Input: dimensioned drawing with shaded views. Units: mm. Origin: part minimum x, y, z. Coordinates: 2 decimals unless noted, no trailing zeros. Order: outer loops, then holes, each group sorted by start corner. A loop starts at its lowest first (then second) coordinate and runs counter-clockwise, first axis right, second up.
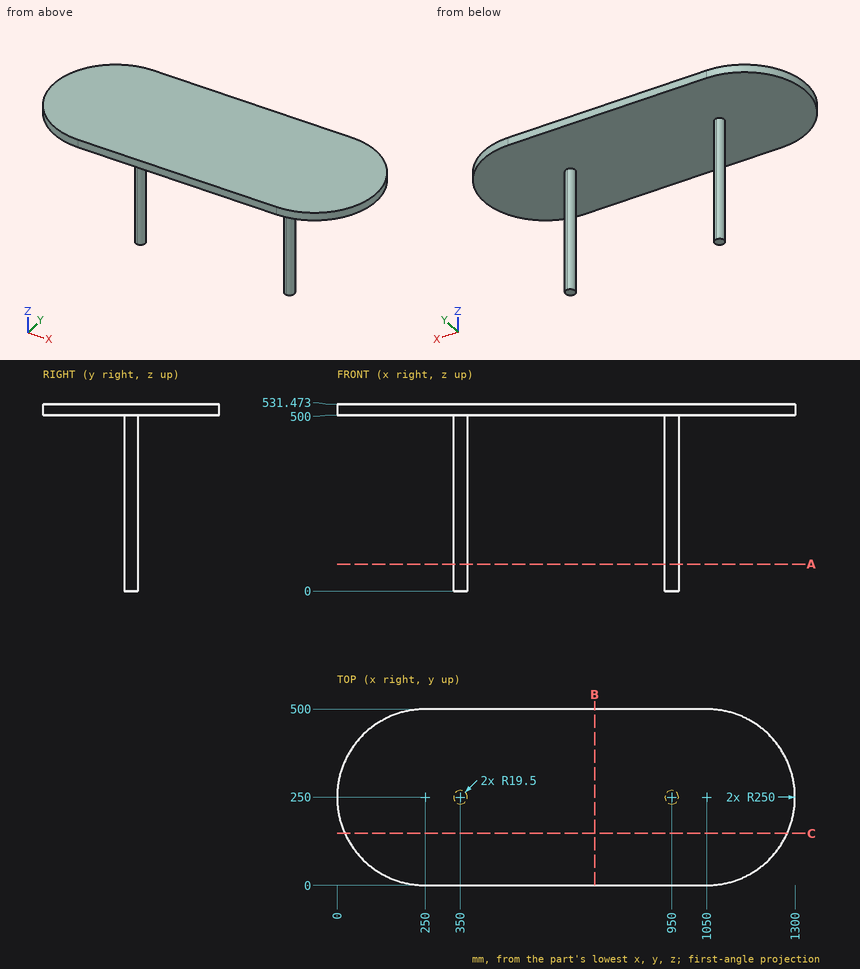
1. Section query B-B, the plane x = 731. Output: boundary loops of the cut face in (y, z).
2. Material intervals for line 1 along X through (y, z) = (252, 384.5); line 2 along Z through (x, y) = (176.5, 88.5); line 3 along X through (y, z) = (233, 219.5), sorted ascending.
3. Section query A-A, the plane z = 76.5. Output: boundary loops of the cut face in (x, y).
4. Section query C-C, the plane y = 147.5. Output: boundary loops of the cut face in (x, z).
Answer key:
1. outline: (0, 500) - (500, 500) - (500, 531.47) - (0, 531.47) - close
2. line 1: x = 330.6 to 369.4, 930.6 to 969.4
2. line 2: z = 500 to 531.47
2. line 3: x = 340.45 to 359.55, 940.45 to 959.55
3. outline: circle Ø39 at (350, 250); circle Ø39 at (950, 250)
4. outline: (21.98, 500) - (1278.02, 500) - (1278.02, 531.47) - (21.98, 531.47) - close
